```python
from build123d import *

# Parameters (mm, degrees)
SKETCH1_W                = 70
SKETCH1_H                = 20
BOSS_EXTRUDE1_DEPTH      = 5
SKETCH2_W                = 90
SKETCH2_H                = 20
BOSS_EXTRUDE2_DEPTH      = 3
BOSS_EXTRUDE3_DEPTH      = 28
CUT_EXTRUDE1_DEPTH       = 59.489315264
FILLET1_R                = 2
FILLET2_R                = 2
M3_CLEARANCE_HOLE1_D     = 3.4
M3_CLEARANCE_HOLE1_DEPTH = 10
M3_CLEARANCE_HOLE1_TIP   = 1.021463052
SKETCH9_W                = 20
SKETCH9_H                = 5
CUT_EXTRUDE2_DEPTH       = 0.3


with BuildPart() as part:
    # Sketch1 → Boss-Extrude1 (new body)
    with BuildSketch(Plane(origin=(0, 0, 0), x_dir=(1, 0, 0), z_dir=(0, 1, 0))):
        Rectangle(SKETCH1_W, SKETCH1_H)
    extrude(amount=BOSS_EXTRUDE1_DEPTH)

    # Sketch2 → Boss-Extrude2 (add)
    with BuildSketch(Plane.XZ):
        Rectangle(SKETCH2_W, SKETCH2_H)
    extrude(amount=BOSS_EXTRUDE2_DEPTH)

    # Sketch4 → Boss-Extrude3 (add)
    with BuildSketch(Plane(origin=(0, 5, 0), x_dir=(1, 0, 0), z_dir=(0, 1, 0))):
        with BuildLine():
            Line((17.5, 10), (-17.5, 10))
            ThreePointArc((-17.5, 10), (0, -7.5), (17.5, 10))
        make_face()
    extrude(amount=BOSS_EXTRUDE3_DEPTH)

    # Sketch6 → Cut-Extrude1 (cut, through all)
    with BuildSketch(Plane(origin=(0, 33, 0), x_dir=(1, 0, 0), z_dir=(0, 1, 0))):
        with BuildLine():
            Line((15.370426149, 8), (-15.370426149, 8))
            ThreePointArc((-15.370426149, 8), (0, -5.5), (15.370426149, 8))
        make_face()
    extrude(amount=-CUT_EXTRUDE1_DEPTH, mode=Mode.SUBTRACT)

    # Fillet1
    fillet1_edges = [part.edges().sort_by_distance(p)[0] for p in [
        (0, 33, 5.5),
        (0, 33, -8),
    ]]
    fillet(fillet1_edges, radius=FILLET1_R - 0.0001)  # a hair under: the kernel refuses the full size

    # Fillet2
    fillet2_edges = [part.edges().sort_by_distance(p)[0] for p in [
        (0, -3, 5.5),
        (0, -3, -8),
    ]]
    fillet(fillet2_edges, radius=FILLET2_R - 0.0001)  # a hair under: the kernel refuses the full size

    # M3 Clearance Hole1
    with Locations(Plane(origin=(0, 0, 0), x_dir=(1, 0, 0), z_dir=(0, 1, 0))):
        with Locations((-40, 6), (-40, -6), (40, 6), (40, -6)):
            Hole(M3_CLEARANCE_HOLE1_D / 2, depth=M3_CLEARANCE_HOLE1_DEPTH)
            with Locations((0, 0, -(M3_CLEARANCE_HOLE1_DEPTH + M3_CLEARANCE_HOLE1_TIP / 2))):  # 118° drill point
                Cone(0, M3_CLEARANCE_HOLE1_D / 2, M3_CLEARANCE_HOLE1_TIP, mode=Mode.SUBTRACT)

    # Sketch9 → Cut-Extrude2 (cut)
    with BuildSketch(Plane.ZY.offset(35)):
        with Locations((0, 2.5)):
            Rectangle(SKETCH9_W, SKETCH9_H)
    extrude(amount=-CUT_EXTRUDE2_DEPTH, mode=Mode.SUBTRACT)


solid = part.part
```
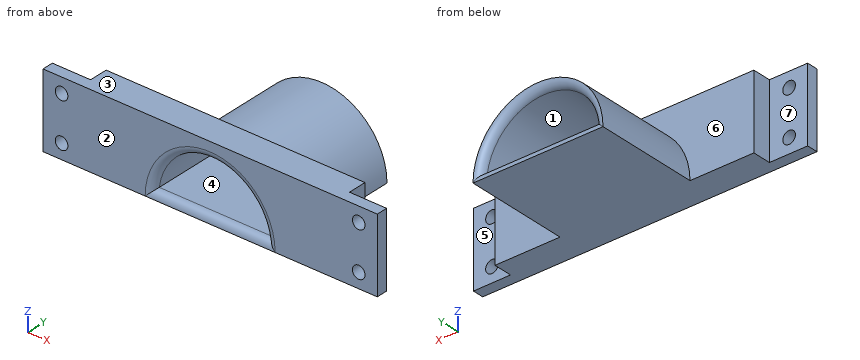
Design review of the part built by this model. Coordinates are the model's own, in mm. Face numbers are marked on the shaded views. A direction names the side the tool comes from. Coordinates: 2 decimals unless noted, no trailing zeros. Order: outer loops, then holes, each group sorted by start corner. A loop starts at its lowest first (then second) coordinate and runs counter-clockwise, first axis right, second up. Notation, with made-up numbers: (-26.75, 54.5) - (19.25, 54.5) arc R27 ccw to (19.25, 79.5) - close; hole circle Ø7 at (70, 42.5). An arc over 180 degrees is marked (long way). Answer in a Markdown table with one row per item.
(1) Consider section D-D on z = -6. Give the number of separate pieces and of enclosed holes in the cut face, plus the area to 3 significant figures.
Checked values:
| item | result |
|---|---|
| separate pieces | 4 |
| enclosed holes | 0 |
| area | 470 mm^2 |
(2) The part is to be moulded in two halves that separate along Z. For the marked faces 1, 2, 3 and 4, say which applies: released by +Z, released by -Z, zero draft, split by the parting line, or undercut.
Checked values:
| item | result |
|---|---|
| face 1 | undercut |
| face 2 | zero draft |
| face 3 | released by +Z |
| face 4 | undercut |
(3) Wall thickness on line 1 along Z through (x, y) = (40, -1); line 2 along X through (y, z) = (-1.5, 6); line 3 along X through (y, z) = (-1, -6): over which ranges is each line inside the solid? List them lowest first. Write a range as from..to.
Checked values:
| item | result |
|---|---|
| line 1 | -10..-7.7, -4.3..4.3, 7.7..10 |
| line 2 | -45..-41.7, -38.3..38.3, 41.7..45 |
| line 3 | -45..-41.7, -38.3..-14.97, 14.97..38.3, 41.7..45 |
(4) Consider section C-C on x = -24. State the section outline as (y, z) points.
Checked values:
| item | result |
|---|---|
| outline | (-3, -10) - (5, -10) - (5, 10) - (-3, 10) - close |
(5) Clearance check with flat-ended pins moving along their axes: pin 1 (3 mm diameter, centred on x = 40.5, z = -4.5, fed in from +Y); pin 2 (2.5 mm diameter, centred on y = 2, z = -4, fed in from -X); pin 3 (4 mm diameter, centred on y = 3.5, z = -1.5, fed in from +X). State where each tip first meets the part, or that it passes through.
Checked values:
| item | result |
|---|---|
| pin 1 | y = 0 |
| pin 2 | x = -34.7 |
| pin 3 | x = 35 |
(6) Consider section A-A on x = -40. State the section outline as (y, z) points, plus the area to 3 significant figures.
Checked values:
| item | result |
|---|---|
| outline | (-3, -10) - (0, -10) - (0, -7.7) - (-3, -7.7) - close; (-3, -4.3) - (0, -4.3) - (0, 4.3) - (-3, 4.3) - close; (-3, 7.7) - (0, 7.7) - (0, 10) - (-3, 10) - close |
| area | 39.6 mm^2 |
(7) For the marked faces 5, 6 and 7, list the 3-axis set-ups (+Z, -Z, +X, -X, +Y, -Y) from which the entire face can be reached by the end or side of a thin tool; tool diameter is ignored.
Checked values:
| item | result |
|---|---|
| face 5 | +Z, -Z, +X, +Y |
| face 6 | +Z, +Y |
| face 7 | +Z, -Z, -X, +Y |
(8) Consider section B-B on y = 23. State the section outline as (x, z) points.
Checked values:
| item | result |
|---|---|
| outline | (-17.5, -10) - (17.5, -10) arc R17.5 ccw to start; hole (-15.37, -8) - (15.37, -8) arc R15.5 ccw to start |
